The model under review builds one solid part; all positions refer to its coordinate system, in mm. Coordinates: 2 decimals unless noted, no trailing zeros. Order: outer loops, then holes, each group sorted by start corner. A loop starts at its lowest first (then second) coordinate and runs counter-clockwise, first axis right, second up.
Autodesk Inventor part; units mm, degrees
ref_plane "YZ Plane" through (0, 0, 0) normal (1, 0, 0) x (0, 1, 0)
ref_plane "XZ Plane" through (0, 0, 0) normal (0, 1, 0) x (-1, 0, 0)
ref_plane "XY Plane" through (0, 0, 0) normal (0, 0, 1) x (1, 0, 0)
sketch "Sketch1" plane through (0, 0, 0) normal (0, 0, 1) x (1, 0, 0)
  line L0 (0, 0) -> (0, 63.5) construction
  line L1 (60, 0) -> (60, 63.5) construction
  line L2 (18, 66.5) -> (42, 66.5) construction
  line L3 (42, 0) -> (18, 0) construction
  circle A0 centre (20, 19.25) radius 1.5
  circle A1 centre (10.45, 31.75) radius 1.35 construction
  circle A2 centre (20, 44.25) radius 1.5
  line L4 (0, 0) -> (60, 0)
  line L5 (60, 0) -> (60, 63.5)
  line L6 (60, 63.5) -> (0, 63.5)
  line L7 (0, 63.5) -> (0, 0)
  circle A3 centre (20, 44.25) radius 1.5
  circle A4 centre (7.5, 31.75) radius 1.5
  circle A5 centre (20, 19.25) radius 1.5
  line L8 (60, 0) -> (42, 0)
  line L9 (60, 0) -> (60, 63.5)
  line L10 (42, 63.5) -> (60, 63.5)
  line L11 (42, 63.5) -> (42, 66.5)
  line L12 (18, 66.5) -> (42, 66.5)
  line L13 (18, 63.5) -> (18, 66.5)
  line L14 (0, 63.5) -> (18, 63.5)
  line L15 (0, 0) -> (0, 63.5)
  line L16 (18, 0) -> (0, 0)
  line L17 (18, 0) -> (18, -3)
  line L18 (18, -3) -> (42, -3)
  line L19 (42, 0) -> (42, -3)
extrude "Extrusion2" add sketch "Sketch1" along normal blind 3 contours L7 L6 L5 L4
properties part number "Pan cross bar spacer"
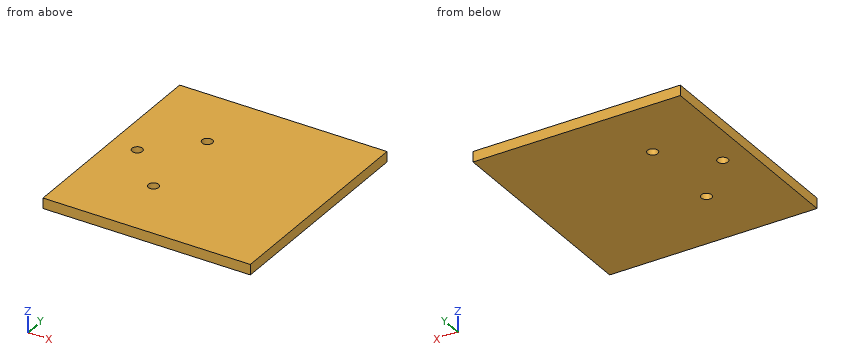
(1) We need section C-C, the plane x = 7.5. Write out the cut boundary in (y, z).
A:
outline: (0, 0) - (30.25, 0) - (30.25, 3) - (0, 3) - close; (33.25, 0) - (63.5, 0) - (63.5, 3) - (33.25, 3) - close
(2) Wall thickness on probe 1 along Y at (x, z) = (20, 2); probe 2 along Y at (x, z) = (7.5, 2.1); probe 3 along X at (y, z) = (44.5, 1.4): over which ranges is each line inside the solid? List them lowest first.
A:
probe 1: y = 0 to 17.75, 20.75 to 42.75, 45.75 to 63.5
probe 2: y = 0 to 30.25, 33.25 to 63.5
probe 3: x = 0 to 18.52, 21.48 to 60
(3) We need section B-B, the plane y = 31.75. Write out the cut boundary in (x, z).
A:
outline: (0, 0) - (6, 0) - (6, 3) - (0, 3) - close; (9, 0) - (60, 0) - (60, 3) - (9, 3) - close
(4) We need section A-A, the plane x = 20. Write out the cut boundary in (y, z).
A:
outline: (0, 0) - (17.75, 0) - (17.75, 3) - (0, 3) - close; (20.75, 0) - (42.75, 0) - (42.75, 3) - (20.75, 3) - close; (45.75, 0) - (63.5, 0) - (63.5, 3) - (45.75, 3) - close
